Geometry: final body of the model. Coordinates: model frame, mm. A direction names the side the tool comes from. Give positions to 0.01 mm unless a question says otherwise; leave off trailing zeros. Write each loop counter-clockwise with the first axis right and the second up, starting at its lowest first coordinate (ties: lowest second). Pieces come first, ordered by that corner, then holes. Notation, with made-up numbers: (86.25, -23) - (125.25, -23) arc R33 cw to (125.25, 8) - close; hole circle Ø9 at (12.25, -17.5). An arc over 180 degrees is marked (long way). Return JSON: item names as keys, results as strings.
from build123d import *

# Parameters (mm, degrees)
EXTRUDE_1_DEPTH                = 5
SKETCH_2_R                     = 6
EXTRUDE_2_DEPTH                = 2.7
CUT_EXTRUDE_1_DEPTH            = 5
SKETCH_4_W                     = 4.5
SKETCH_4_H                     = 0.5
HOLE_WIZARD_M2_5_1_D           = 3
HOLE_WIZARD_M2_5_1_DEPTH       = 8.2
HOLE_WIZARD_M2_5_1_CBORE_D     = 6.8
HOLE_WIZARD_M2_5_1_CBORE_DEPTH = 2.9


with BuildPart() as part:
    # 스케치1 → 보스-돌출1 (new body)
    with BuildSketch(Plane(origin=(0, 0, 0), x_dir=(-1, 0, 0), z_dir=(0, 0, -1))):
        with BuildLine():
            Line((0, -7.5), (-35, -7.5))
            ThreePointArc((-35, -7.5), (-42.5, 0), (-35, 7.5))
            Line((-35, 7.5), (0, 7.5))
            ThreePointArc((0, 7.5), (7.5, 0), (0, -7.5))
        make_face()
    extrude(amount=-EXTRUDE_1_DEPTH)

    # 스케치2 → 보스-돌출2 (add)
    with BuildSketch(Plane(origin=(0, 0, 0), x_dir=(-1, 0, 0), z_dir=(0, 0, -1))):
        with Locations(Location((0, 0, 0), (0, 0, 180))):
            Circle(SKETCH_2_R)
    extrude(amount=EXTRUDE_2_DEPTH)

    # 스케치3 → 컷-돌출1 (cut)
    with BuildSketch(Plane(origin=(0, 0, -2.7), x_dir=(-1, 0, 0), z_dir=(0, 0, -1))):
        with BuildLine():
            Line((-0.820496547, 3.65913725), (-1.32189409, 2.969022737))
            Line((-1.32189409, 2.969022737), (-2.170249561, 3.05818849))
            ThreePointArc((-2.170249561, 3.05818849), (-2.204194696, 3.033813729), (-2.237866095, 3.009062203))
            Line((-2.237866095, 3.009062203), (-2.415220683, 2.174674471))
            Line((-2.415220683, 2.174674471), (-3.226498949, 1.911074183))
            ThreePointArc((-3.226498949, 1.911074183), (-3.247595264, 1.875), (-3.268288265, 1.838692964))
            Line((-3.268288265, 1.838692964), (-3.090933678, 1.004305232))
            Line((-3.090933678, 1.004305232), (-3.724857357, 0.433517788))
            ThreePointArc((-3.724857357, 0.433517788), (-3.729457108, 0.391981737), (-3.733593703, 0.350397007))
            Line((-3.733593703, 0.350397007), (-3.23219616, -0.339717506))
            Line((-3.23219616, -0.339717506), (-3.579154088, -1.118997772))
            ThreePointArc((-3.579154088, -1.118997772), (-3.566461936, -1.158813729), (-3.55332687, -1.198485775))
            Line((-3.55332687, -1.198485775), (-2.814582562, -1.625))
            Line((-2.814582562, -1.625), (-2.814582562, -2.47802845))
            ThreePointArc((-2.814582562, -2.47802845), (-2.786793096, -2.509239774), (-2.758657541, -2.540139479))
            Line((-2.758657541, -2.540139479), (-1.91030207, -2.629305232))
            Line((-1.91030207, -2.629305232), (-1.563344142, -3.408585498))
            ThreePointArc((-1.563344142, -3.408585498), (-1.525262412, -3.425795466), (-1.486991261, -3.44257999))
            Line((-1.486991261, -3.44257999), (-0.675712995, -3.178979702))
            Line((-0.675712995, -3.178979702), (-0.041789316, -3.749767147))
            ThreePointArc((-0.041789316, -3.749767147), (0, -3.75), (0.041789316, -3.749767147))
            Line((0.041789316, -3.749767147), (0.675712995, -3.178979702))
            Line((0.675712995, -3.178979702), (1.486991261, -3.44257999))
            ThreePointArc((1.486991261, -3.44257999), (1.525262412, -3.425795466), (1.563344142, -3.408585498))
            Line((1.563344142, -3.408585498), (1.91030207, -2.629305232))
            Line((1.91030207, -2.629305232), (2.758657541, -2.540139479))
            ThreePointArc((2.758657541, -2.540139479), (2.786793096, -2.509239774), (2.814582562, -2.47802845))
            Line((2.814582562, -2.47802845), (2.814582562, -1.625))
            Line((2.814582562, -1.625), (3.55332687, -1.198485775))
            ThreePointArc((3.55332687, -1.198485775), (3.566461936, -1.158813729), (3.579154088, -1.118997772))
            Line((3.579154088, -1.118997772), (3.23219616, -0.339717506))
            Line((3.23219616, -0.339717506), (3.733593703, 0.350397007))
            ThreePointArc((3.733593703, 0.350397007), (3.729457108, 0.391981737), (3.724857357, 0.433517788))
            Line((3.724857357, 0.433517788), (3.090933678, 1.004305232))
            Line((3.090933678, 1.004305232), (3.268288265, 1.838692964))
            ThreePointArc((3.268288265, 1.838692964), (3.247595264, 1.875), (3.226498949, 1.911074183))
            Line((3.226498949, 1.911074183), (2.415220683, 2.174674471))
            Line((2.415220683, 2.174674471), (2.237866095, 3.009062203))
            ThreePointArc((2.237866095, 3.009062203), (2.204194696, 3.033813729), (2.170249561, 3.05818849))
            Line((2.170249561, 3.05818849), (1.32189409, 2.969022737))
            Line((1.32189409, 2.969022737), (0.820496547, 3.65913725))
            ThreePointArc((0.820496547, 3.65913725), (0.779668841, 3.668053503), (0.738744308, 3.676514225))
            Line((0.738744308, 3.676514225), (0, 3.25))
            Line((0, 3.25), (-0.738744308, 3.676514225))
            ThreePointArc((-0.738744308, 3.676514225), (-0.779668841, 3.668053503), (-0.820496547, 3.65913725))
        make_face()
    extrude(amount=-CUT_EXTRUDE_1_DEPTH, mode=Mode.SUBTRACT)

    # 스케치4 → 회전1 (revolve)
    with BuildSketch(Plane.XZ, mode=Mode.PRIVATE) as revolve_1_sk:
        with Locations((2.25, 5.25)):
            Rectangle(SKETCH_4_W, SKETCH_4_H)
    revolve(revolve_1_sk.sketch.rotate(Axis((0, 0, 5.5), (0, 0, -1)), 180), axis=Axis((0, 0, 5.5), (0, 0, -1)))

    # M2.5 육각 머리 작은 나사용 카운터보어1
    with Locations(Plane.XY.offset(5.5)):
        with Locations((0, 0)):
            CounterBoreHole(HOLE_WIZARD_M2_5_1_D / 2, HOLE_WIZARD_M2_5_1_CBORE_D / 2, HOLE_WIZARD_M2_5_1_CBORE_DEPTH, depth=HOLE_WIZARD_M2_5_1_DEPTH)


solid = part.part
Q1. Section query A-A, the plane y = 5. Return the cut outline in (x, z).
Answer key:
{"outline": "(-5.59, 0) - (-3.32, 0) - (-3.32, -2.7) - (3.32, -2.7) - (3.32, 0) - (40.59, 0) - (40.59, 5) - (-5.59, 5) - close"}
Q2. Material intervals for probe 1 along Y at (x, z) = (0, 2.5); probe 2 along X at (y, z) = (-0.25, 4.5); probe 3 along Z at (x, y) = (16, 1.25), sorted ascending. Write a range as [from, to].
Answer key:
{"probe 1": "y = [-7.5, -1.5], [1.5, 7.5]", "probe 2": "x = [-7.5, -3.39], [3.39, 42.5]", "probe 3": "z = [0, 5]"}
Q3. Pin query (flat end, axial travel): P1, Ø3, axis at x = -1, z = 0, coming from the -Y side; P2, Ø4, axis at x = 0, y = 0, coming from the -Z side; P3, Ø0.7, axis at y = -2, z = 0.5, coming from the +X side. Return the tip coordinate at first contact, or that it passes through.
Answer key:
{"P1": "stops at y = -7.5", "P2": "stops at z = 2.3", "P3": "stops at x = 42.32"}
Q4. Set-up query: faces 4 (the flat face through (0, -2, 2.3)), 5 (the flat face through (1.5, -0.7, 2.6)), 6 (the cylindrical face through (-7.5, 0.16, 2.46)). Return all of +Z, -Z, +X, -X, +Y, -Y with unobstructed straight access to the full face (end or side cutting, diameter ignored); none if empty.
Answer key:
{"face 4": "-Z", "face 5": "+Z", "face 6": "+Z, -Z, -X"}
Q5. Section query B-B, the plane x = 22. Return the cut outline in (y, z), plus the area to 3 significant figures.
Answer key:
{"outline": "(-7.5, 0) - (7.5, 0) - (7.5, 5) - (-7.5, 5) - close", "area": "75.0 mm^2"}
Q6. Mould query, pull axis Y, two halves, no side actions, for faces 1 (the flat face through (2.815, 2.045, -0.235)), 2 (the cylindrical face through (42.5, -0.16, 2.46)), 3 (the flat face through (17, 0, 5)). Classes: pulls with the +Y half, pulls with the -Y half, needs draft (parallel to the pull), parting line crosses it, or undercut.
Answer key:
{"face 1": "undercut", "face 2": "parting line crosses it", "face 3": "needs draft"}
